from build123d import *

# Parameters (mm, degrees)
SKETCH_1_R               = 17.5
EXTRUDE_1_DEPTH          = 11
SKETCH_2_R               = 1.5
CUT_EXTRUDE_1_DEPTH      = 5
PATTERN_CIRCULAR_1_COUNT = 6
SKETCH_3_R               = 3
CUT_EXTRUDE_2_DEPTH      = 3
SKETCH_4_R               = 1.5
CUT_EXTRUDE_3_DEPTH      = 5


with BuildPart() as part:
    # 草图1 → 凸台-拉伸1 (new body)
    with BuildSketch(Plane.XY):
        Circle(SKETCH_1_R)
    extrude(amount=EXTRUDE_1_DEPTH)

    # 草图2 → 切除-拉伸1 (cut)
    with BuildSketch(Plane.XY.offset(11)):
        with Locations((13.5, 0)):
            Circle(SKETCH_2_R)
    cut_extrude_1 = extrude(amount=-CUT_EXTRUDE_1_DEPTH, mode=Mode.SUBTRACT)

    # 阵列(圆周)1: 切除-拉伸1 ×6 about axis
    pattern_circular_1_axis = Axis((0, 0, 0), (0, 0, 1))
    for i in range(1, PATTERN_CIRCULAR_1_COUNT):
        add(cut_extrude_1.rotate(pattern_circular_1_axis, i * 360 / PATTERN_CIRCULAR_1_COUNT), mode=Mode.SUBTRACT)

    # 草图3 → 切除-拉伸2 (cut)
    with BuildSketch(Plane.XY.offset(11)):
        Circle(SKETCH_3_R)
    extrude(amount=-CUT_EXTRUDE_2_DEPTH, mode=Mode.SUBTRACT)

    # 草图4 → 切除-拉伸3 (cut)
    with BuildSketch(Plane.XY.offset(8)):
        Circle(SKETCH_4_R)
    extrude(amount=-CUT_EXTRUDE_3_DEPTH, mode=Mode.SUBTRACT)


solid = part.part
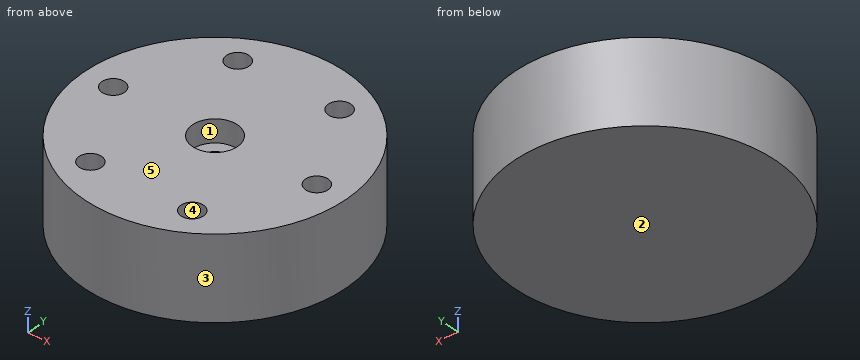
Verification items for the finished model (mm, model axes). Face numbers are marked on the shaded views. A direction names the side the tool comes from. Round coordinates to 2 decimals unless told otherwise and drop trailing zeros. Loops run counter-clockwise (first coordinate to the right, second up) from the corner with the lowest first, then second, coordinate; pieces in that order, holes last. Notation, with made-up numbers: (-29.5, 58) - (-17.5, 58) arc R32 ccw to (-17.5, 86) - close; hole circle Ø6 at (77.5, 60). An arc over 180 degrees is marked (long way). Use a Markdown table: item, result. Add a question column.
1. Release check for a two-part mould opening along X. For the marked faces 1, 2 and 3 record: released by +X, released by -X, zero draft, split by the parting line, or undercut.
2. Gauge pin test, flat ends, axial feed: pin 1 (0.9 mm diameter, centred on x = 13, y = 0.5, fed in from +Z); pin 2 (5 mm diameter, centred on x = -4, z = 3, fed in from +Y); pin 3 (4 mm diameter, centred on y = 4, z = 7.5, fed in from -X). Record the tip position at first contact, or that the pin passes through.
3. Section check A-A, the plane z = 6.75. Record the boundary of the cut face in (x, y).
4. Section check B-B, the plane x = 12.5. Record the boundary of the cut face in (y, z), plus the area to 3 significant figures.
5. Section check C-C, the plane y = 0. Record the boundary of the cut face in (x, z), plus the area to 3 significant figures.
6. Access from +Z, -Z, +X, -X, +Y, -Y to the whole of each face (thin tool, end or side, straight path). Record for the marked faces 4 and 5.
7. Thickness scan on probe 1 along X at (y, z) = (11, 10.5); probe 2 along X at (y, z) = (-13, 7.25); probe 3 along X at (y, z) = (11.5, 2.5). Record the ranges inside material, lowest first. Write a range as [from, to].
8. Section check D-D, the plane z = 4.25. Record the boundary of the cut face in (x, y), plus the area to 3 significant figures.
Checks:
| question | item | result |
|---|---|---|
| 1 | face 1 | undercut |
| 1 | face 2 | zero draft |
| 1 | face 3 | split by the parting line |
| 2 | pin 1 | stops at z = 6 |
| 2 | pin 2 | stops at y = 17.44 |
| 2 | pin 3 | stops at x = -17.39 |
| 3 | outline | circle Ø35 at (0, 0); hole circle Ø3 at (-13.5, 0); hole circle Ø3 at (-6.75, -11.69); hole circle Ø3 at (-6.75, 11.69); hole circle Ø3 at (0, 0); hole circle Ø3 at (6.75, -11.69); hole circle Ø3 at (6.75, 11.69); hole circle Ø3 at (13.5, 0) |
| 4 | outline | (-12.25, 0) - (12.25, 0) - (12.25, 11) - (1.12, 11) - (1.12, 6) - (-1.12, 6) - (-1.12, 11) - (-12.25, 11) - close |
| 4 | area | 258 mm^2 |
| 5 | outline | (-17.5, 0) - (17.5, 0) - (17.5, 11) - (15, 11) - (15, 6) - (12, 6) - (12, 11) - (3, 11) - (3, 8) - (1.5, 8) - (1.5, 3) - (-1.5, 3) - (-1.5, 8) - (-3, 8) - (-3, 11) - (-12, 11) - (-12, 6) - (-15, 6) - (-15, 11) - (-17.5, 11) - close |
| 5 | area | 322 mm^2 |
| 6 | face 4 | +Z |
| 6 | face 5 | +Z, +X, -X, +Y, -Y |
| 7 | probe 1 | x = [-13.61, -8.08], [-5.42, 5.42], [8.08, 13.61] |
| 7 | probe 2 | x = [-11.72, -7.48], [-6.02, 6.02], [7.48, 11.72] |
| 7 | probe 3 | x = [-13.19, 13.19] |
| 8 | outline | circle Ø35 at (0, 0); hole circle Ø3 at (0, 0) |
| 8 | area | 955 mm^2 |
